Build history of the part. All positions in model axes, mm. Round coordinates to 2 decimals unless told otherwise and drop trailing zeros. Write each loop counter-clockwise with the first axis right and the second up, starting at its lowest first coordinate (ties: lowest second). Pieces come first, ordered by that corner, then holes. Notation, with made-up numbers: (65, 23) - (76, 23) arc R23 ccw to (76, 46) - close; hole circle Ø11 at (43.5, 19.25). An arc over 180 degrees is marked (long way). One line per question, with ' | ' between items.
from build123d import *

# Parameters (mm, degrees)
BOSS_EXTRUDE1_DEPTH = 3
ESBO_O1_R           = 3.05
ESBO_O1_R_2         = 3.55
ESBO_O1_R_3         = 4.05
ESBO_O1_R_4         = 1.55
CUT_EXTRUDE2_DEPTH  = 10


# Read off the part's stored shape, not the designer's step: Boss-Extrude1
with BuildPart() as part:
    # Boss-Extrude1 outline → Boss-Extrude1 (new body)
    with BuildSketch(Plane.XY):
        Polygon((0, 0), (-0.86472917, -16.500015494), (0, -33.000030988), (130.305174389, -32.999992472), (131.13382584, -15.81161159), (130.305174389, 0), align=None)
    extrude(amount=BOSS_EXTRUDE1_DEPTH)

    # Esboço1 → Cut-Extrude2 (cut)
    with BuildSketch(Plane.XY.offset(3)):
        with Locations((15.264794979, -16.500000001)):
            Circle(ESBO_O1_R)
        with Locations((29.34491573, -16.500000001)):
            Circle(ESBO_O1_R_2)
        with Locations((43.432199078, -16.500000001)):
            Circle(ESBO_O1_R_3)
        with Locations((57.519151999, -16.500000001)):
            Circle(ESBO_O1_R_3)
        with Locations((71.597045458, -16.500000001)):
            Circle(ESBO_O1_R_3)
        with Locations((86.59615234, -2.1587967)):
            Circle(ESBO_O1_R_4)
        with Locations((116.99615234, -2.1587967)):
            Circle(ESBO_O1_R_4)
        with Locations((86.59615234, -30.8412033)):
            Circle(ESBO_O1_R_4)
        with Locations((116.99615234, -30.8412033)):
            Circle(ESBO_O1_R_4)
    extrude(amount=-CUT_EXTRUDE2_DEPTH, mode=Mode.SUBTRACT)


solid = part.part
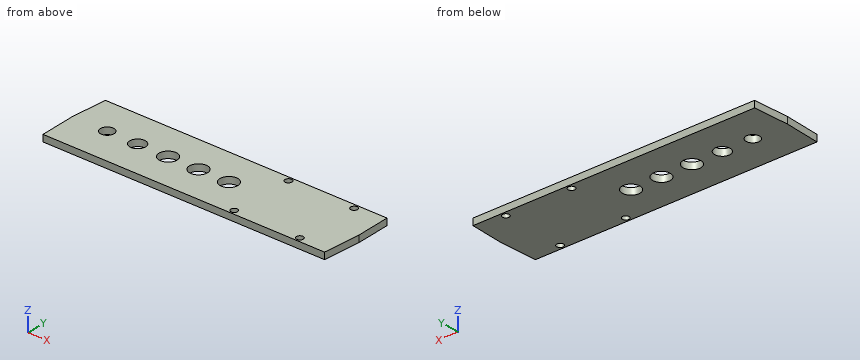
Q1. Drill centre lines: L1, parallel to X at y = -17, z = 1.65; L2, parallel to X at y = -16.5, z = 0.95; L3, parallel to Y at x = 73.5, z = 2.3. Where is each one in solid material? Low to high. Write a range as from..to.
Found:
L1: -0.84..12.26, 18.27..25.83, 32.86..39.41, 47.45..53.5, 61.54..67.58, 75.62..131.08 | L2: -0.86..12.21, 18.31..25.79, 32.89..39.38, 47.48..53.47, 61.57..67.55, 75.65..131.1 | L3: -33..-20.08, -12.92..0
Q2. Drop flat-ended pins along their axis: pin 1 (3 mm diameter, centred on x = 117, y = -30.84, fed in from +Z); pin 2 (1 mm diameter, centred on y = -25.5, z = 2.5, fed in from -X). Give the stop position or say it passes through.
Found:
pin 1: through | pin 2: x = -0.42
Q3. Saw through at A-A, the plane x = 44.5. List the corners of the cut face in (y, z).
Found:
outline: (-33, 0) - (-20.41, 0) - (-20.41, 3) - (-33, 3) - close; (-12.59, 0) - (0, 0) - (0, 3) - (-12.59, 3) - close
